from build123d import *

# Parameters (mm, degrees)
SKETCH2_R           = 11.1125
SKETCH2_R_2         = 2.4892
SKETCH2_R_3         = 22.225
BOSS_EXTRUDE1_DEPTH = 3.175


with BuildPart() as part:
    # Sketch2 → Boss-Extrude1 (new body)
    with BuildSketch(Plane.XY):
        with BuildLine():
            Line((142.632381685, 122.462939957), (142.632381685, -29.937060043))
            ThreePointArc((142.632381685, -29.937060043), (116.6794163, -47.687448689), (106.68, -77.497587619))
            Line((106.68, -77.497587619), (106.68, -128.297587619))
            Line((106.68, -128.297587619), (96.52, -128.297587619))
            ThreePointArc((96.52, -128.297587619), (85.109838908, -95.769716492), (55.88, -77.497587619))
            Line((55.88, -77.497587619), (-55.88, -77.497587619))
            ThreePointArc((-55.88, -77.497587619), (-85.109838908, -95.769716492), (-96.52, -128.297587619))
            Line((-96.52, -128.297587619), (-106.68, -128.297587619))
            Line((-106.68, -128.297587619), (-106.68, -77.497587619))
            ThreePointArc((-106.68, -77.497587619), (-116.6794163, -47.687448689), (-142.632381685, -29.937060043))
            Line((-142.632381685, -29.937060043), (-142.632381685, 122.462939957))
            ThreePointArc((-142.632381685, 122.462939957), (-134.600001748, 148.101160684), (-108.918256202, 140.209048469))
            Line((-108.918256202, 140.209048469), (-31.75, 0))
            ThreePointArc((-31.75, 0), (0, -31.75), (31.75, 0))
            Line((31.75, 0), (108.918256202, 140.209048468))
            ThreePointArc((108.918256202, 140.209048468), (134.600001748, 148.101160684), (142.632381685, 122.462939957))
        make_face()
        with Locations((-60.484532313, 12.7)):
            Circle(SKETCH2_R, mode=Mode.SUBTRACT)
        with Locations((-125.726814921, 131.243846084)):
            Circle(SKETCH2_R, mode=Mode.SUBTRACT)
        with Locations((125.726814921, 131.243846084)):
            Circle(SKETCH2_R, mode=Mode.SUBTRACT)
        with Locations((-101.9175, -57.15)):
            Circle(SKETCH2_R_2, mode=Mode.SUBTRACT)
        with Locations((60.484532313, 12.7)):
            Circle(SKETCH2_R, mode=Mode.SUBTRACT)
        with Locations((-89.2175, -57.15)):
            Circle(SKETCH2_R_2, mode=Mode.SUBTRACT)
        with Locations((-76.5175, -57.15)):
            Circle(SKETCH2_R_2, mode=Mode.SUBTRACT)
        with Locations((-63.8175, -57.15)):
            Circle(SKETCH2_R_2, mode=Mode.SUBTRACT)
        with Locations((-51.1175, -57.15)):
            Circle(SKETCH2_R_2, mode=Mode.SUBTRACT)
        with Locations((-38.4175, -57.15)):
            Circle(SKETCH2_R_2, mode=Mode.SUBTRACT)
        with Locations((-25.7175, -57.15)):
            Circle(SKETCH2_R_2, mode=Mode.SUBTRACT)
        with Locations((-13.0175, -57.15)):
            Circle(SKETCH2_R_2, mode=Mode.SUBTRACT)
        with Locations((-0.3175, -57.15)):
            Circle(SKETCH2_R_2, mode=Mode.SUBTRACT)
        with Locations((12.3825, -57.15)):
            Circle(SKETCH2_R_2, mode=Mode.SUBTRACT)
        with Locations((25.0825, -57.15)):
            Circle(SKETCH2_R_2, mode=Mode.SUBTRACT)
        with Locations((37.7825, -57.15)):
            Circle(SKETCH2_R_2, mode=Mode.SUBTRACT)
        with Locations((50.4825, -57.15)):
            Circle(SKETCH2_R_2, mode=Mode.SUBTRACT)
        with Locations((63.1825, -57.15)):
            Circle(SKETCH2_R_2, mode=Mode.SUBTRACT)
        with Locations((75.8825, -57.15)):
            Circle(SKETCH2_R_2, mode=Mode.SUBTRACT)
        with Locations((88.5825, -57.15)):
            Circle(SKETCH2_R_2, mode=Mode.SUBTRACT)
        with Locations((101.2825, -57.15)):
            Circle(SKETCH2_R_2, mode=Mode.SUBTRACT)
        with Locations((-101.9175, -69.85)):
            Circle(SKETCH2_R_2, mode=Mode.SUBTRACT)
        with Locations((-101.9175, -82.55)):
            Circle(SKETCH2_R_2, mode=Mode.SUBTRACT)
        with Locations((-101.9175, -95.25)):
            Circle(SKETCH2_R_2, mode=Mode.SUBTRACT)
        with Locations((-101.9175, -107.95)):
            Circle(SKETCH2_R_2, mode=Mode.SUBTRACT)
        with Locations((-101.9175, -120.65)):
            Circle(SKETCH2_R_2, mode=Mode.SUBTRACT)
        with Locations((101.2825, -69.85)):
            Circle(SKETCH2_R_2, mode=Mode.SUBTRACT)
        with Locations((101.2825, -82.55)):
            Circle(SKETCH2_R_2, mode=Mode.SUBTRACT)
        with Locations((101.2825, -95.25)):
            Circle(SKETCH2_R_2, mode=Mode.SUBTRACT)
        with Locations((101.2825, -107.95)):
            Circle(SKETCH2_R_2, mode=Mode.SUBTRACT)
        with Locations((101.2825, -120.65)):
            Circle(SKETCH2_R_2, mode=Mode.SUBTRACT)
        with Locations((-106.68, -9.525)):
            Circle(SKETCH2_R_3, mode=Mode.SUBTRACT)
        with Locations((106.68, -9.525)):
            Circle(SKETCH2_R_3, mode=Mode.SUBTRACT)
    extrude(amount=BOSS_EXTRUDE1_DEPTH)


solid = part.part
Can you work these out from the model? Positions are in its coordinate system, mm. A direction names the side the tool comes from. Coordinates: 2 decimals unless noted, no trailing zeros. Loops run counter-clockwise (first coordinate to the right, second up) from the corner with the lowest first, then second, coordinate; pieces in that order, holes last. Notation, with made-up numbers: (-19, -16.5) - (14, -16.5) arc R13 ccw to (14, 1.5) - close; hole circle Ø5 at (21.5, 43.5). An arc over 180 degrees is marked (long way). Put each result on its own line as item: value. Start each with the question number.
Item 1: Suppose I cut it at A-A (y = -15). Please give me the cut outline in (x, z) (3 decimals), and give its area (3 significant figures).
Item 2: If we mould it in two halves opening along Y, with no side actions, what happens to faces 1 (the face through (-71.586, 13.189, 1.565)), 2 (the face through (117.536, 138.754, 1.565)), 3 (the face through (85.42, -96.16, 1.57)), 4 (the face through (134.23, 148.29, 1.57))? For each: +Y half, -Y half, draft (parallel to the pull), parting line (faces both ways), or undercut.
Item 3: For pin 1 (3 mm diameter, centred on x = 101.28, y = -82.55, fed in from -Z); pin 2 (1 mm diameter, centred on y = -3, z = 2.5, fed in from +X), each with a flat end and sliding along its axis, tell me the tip position at first contact or that it passes through.
Item 4: If I drill on line 1 along X through (y, z) = (-106, 2.5); line 2 along Y through (x, z) = (-116, 2.25); line 3 along X through (y, z) = (-3.5, 1.5), over which ranges is the centre line in solid material (lowest first)?
Item 5: Which directions (+Z, -Z, +X, -X, +Y, -Y) give clear straight access to the entire face, cutting with the end or side of a thin tool? Please do faces 5 (the face through (-84.801, -95.387, 1.565)), 6 (the face through (-70.874, 71.086, 1.565)), 7 (the face through (-116.41, -48.05, 1.57)).
Item 6: Suppose I cut it at C-C (z = 2.3). State how many separate pieces and enclosed holes the cut face has, and give its area (3 significant figures).
Item 7: Suppose I cut it at B-B (y = 38.5). Please give me the cut outline in (x, z) (3 decimals).
Here are the results:
1. outline: (-142.632, 0) - (-128.22, 0) - (-128.22, 3.175) - (-142.632, 3.175) - close; (-85.14, 0) - (-27.983, 0) - (-27.983, 3.175) - (-85.14, 3.175) - close; (27.983, 0) - (85.14, 0) - (85.14, 3.175) - (27.983, 3.175) - close; (128.22, 0) - (142.632, 0) - (142.632, 3.175) - (128.22, 3.175) - close
1. area: 454 mm²
2. face 1: undercut
2. face 2: undercut
2. face 3: -Y half
2. face 4: parting line
3. pin 1: through
3. pin 2: x = 142.63
4. line 1: -106.68 to -103.46, -100.37 to -91.5, 91.5 to 99.74, 102.83 to 106.68
4. line 2: -48.61 to -29.7, 10.65 to 125.87, 136.62 to 147.62
4. line 3: -142.63 to -128.07, -85.29 to -31.56, 31.56 to 85.29, 128.07 to 142.63
5. face 5: +Z, -Z, -Y
5. face 6: +Z, -Z, +Y
5. face 7: +Z, -Z, -X, -Y
6. separate pieces: 1
6. enclosed holes: 33
6. area: 35,700 mm²
7. outline: (-142.632, 0) - (-52.94, 0) - (-52.94, 3.175) - (-142.632, 3.175) - close; (52.94, 0) - (142.632, 0) - (142.632, 3.175) - (52.94, 3.175) - close
